```python
from build123d import *

# Parameters (mm, degrees)
F1_W     = 58
F1_H     = 48
F1_W_2   = 50
F1_H_2   = 40
F2_DEPTH = 4
F3_SIZE2 = 3.59999
F3_SIZE  = 3.99999


# Not quite as in the source:
# - a fillet or chamfer is up to 0.001 mm smaller than in the source, because OpenCascade refuses the exact size


with BuildPart() as f2:
    # F1 (on Front) → F2 (new body)
    with BuildSketch(Plane.XZ):
        Rectangle(F1_W, F1_H)
        Rectangle(F1_W_2, F1_H_2, mode=Mode.SUBTRACT)
    extrude(amount=F2_DEPTH)

    # F3 (size 4 and 3.6 in the source; OpenCascade refuses exactly that, so slightly less here)
    f3_edges = [f2.edges().sort_by_distance(p)[0] for p in [
        (-25, -4, 0),
        (0, -4, 20),
        (25, -4, 0),
        (0, -4, -20),
    ]]
    f3_side = f2.faces().sort_by_distance((28.247139, -4, 0))[0]
    chamfer(f3_edges, length=F3_SIZE, length2=F3_SIZE2, reference=f3_side)


solid = f2.part
```
For this review, take the finished solid that the model builds, in its own axes (mm). A direction names the side the tool comes from. Give positions to 0.01 mm unless a question says otherwise; leave off trailing zeros. Loops run counter-clockwise (first coordinate to the right, second up) from the corner with the lowest first, then second, coordinate; pieces in that order, holes last. Notation, with made-up numbers: M 44.25,-30 L 99.25,-30 A10 cw 99.25,-16 Z; hole C 21.5,64.25 d8. An arc over 180 degrees is marked long. One line per item, written item: value. Start each with the question number.
Q1. Clearance check with flat-ended pins moving along their axes: pin 1 Ø12 at (x, z) = (6.5, 14.5) entering from +Y; pin 2 Ø6 at (x, z) = (-0.5, -16) entering from +Y. State where each tip first meets the part, or that it passes through.
Q2. Machinability: for faces 4 (the face through (-27, -2.2, -0.3)), 5 (the face through (0, 0, -21)), which of the approach directions +Z, -Z, +X, -X, +Y, -Y give a long, thin tool a straight path to every point of the face, cutting with its end or side? Answer none if there is none.
Q3. For L1, parallel to Z at x = 10.5, y = -0.2; L2, parallel to X at y = -0.5, z = -6; L3, parallel to Z at x = 15, y = -3.35, list the stretches that pass through material, from the lowest coordinate up.
Q4. Add section C-C (y = -2.1). Give the boundary of the cut face in (x, z).
Q5. Draft analysis for pull direction X (two halves, no side actions). For faces 1 (the face through (29, -2, 0)), 2 (the face through (27, -2.2, -0.3)), 3 (the face through (0, -2, 24)), state which applies: released by +X, released by -X, zero draft, split by the parting line, or undercut.
Reply:
1. pin 1: y = 0
1. pin 2: through
2. face 4: -Y
2. face 5: +Z, -Z, +X, -X, +Y
3. L1: -24 to -20, 20 to 24
3. L2: -29 to -25.11, 25.11 to 29
3. L3: -24 to -23.28, 23.28 to 24
4. outline: M -29,-24 L 29,-24 L 29,24 L -29,24 Z; hole M -26.89,-21.89 L 26.89,-21.89 L 26.89,21.89 L -26.89,21.89 Z
5. face 1: released by +X
5. face 2: undercut
5. face 3: zero draft
